from build123d import *

# Parameters (mm, degrees)
SKETCH_1_W          = 60
SKETCH_1_H          = 32
EXTRUDE_1_DEPTH     = 180
SKETCH_2_W          = 56
SKETCH_2_H          = 26
CUT_EXTRUDE_1_DEPTH = 30


with BuildPart() as part:
    # 草图1 → 凸台-拉伸1 (new body)
    with BuildSketch(Plane.XY):
        with Locations((30, 16)):
            Rectangle(SKETCH_1_W, SKETCH_1_H)
    extrude(amount=EXTRUDE_1_DEPTH)

    # 草图2 → 切除-拉伸1 (cut)
    with BuildSketch(Plane(origin=(0, 0, 0), x_dir=(-1, 0, 0), z_dir=(0, -1, 0))):
        with Locations((-30, -165)):
            Rectangle(SKETCH_2_W, SKETCH_2_H)
        with Locations((-30, -135.5)):
            Rectangle(SKETCH_2_W, SKETCH_2_H)
        with Locations((-30, -106)):
            Rectangle(SKETCH_2_W, SKETCH_2_H)
        with Locations((-30, -76.5)):
            Rectangle(SKETCH_2_W, SKETCH_2_H)
        with Locations((-30, -47)):
            Rectangle(SKETCH_2_W, SKETCH_2_H)
        with Locations((-30, -17.5)):
            Rectangle(SKETCH_2_W, SKETCH_2_H)
    extrude(amount=-CUT_EXTRUDE_1_DEPTH, mode=Mode.SUBTRACT)


solid = part.part
Build history of the part. All positions in model axes, mm. A direction names the side the tool comes from. Give positions to 0.01 mm unless a question says otherwise; leave off trailing zeros. Order: outer loops, then holes, each group sorted by start corner. A loop starts at its lowest first (then second) coordinate and runs counter-clockwise, first axis right, second up. Notation, with made-up numbers: M 48.25,46 L 60.25,46 A34 ccw 60.25,84 Z; hole C 1.5,2 d1. An arc over 180 degrees is marked long. Put each result on its own line as item: value.
Item 1: Cut at C-C on x = 13. Write the cut outline in (y, z), then the cut area to 3 significant figures.
Results are:
outline: M 0,0 L 32,0 L 32,180 L 0,180 L 0,178 L 30,178 L 30,152 L 0,152 L 0,148.5 L 30,148.5 L 30,122.5 L 0,122.5 L 0,119 L 30,119 L 30,93 L 0,93 L 0,89.5 L 30,89.5 L 30,63.5 L 0,63.5 L 0,60 L 30,60 L 30,34 L 0,34 L 0,30.5 L 30,30.5 L 30,4.5 L 0,4.5 Z
area: 1,080 mm2
Item 2: Cut at A-A on z = 162. Write the cut outline in (x, y).
Results are:
outline: M 0,0 L 2,0 L 2,30 L 58,30 L 58,0 L 60,0 L 60,32 L 0,32 Z
Item 3: Drop flat-ended pins along their axis: pin 1 Ø6 at (x, y) = (17.5, 7.5) entering from -Z; pin 2 Ø21 at (x, z) = (19.5, 107) entering from -Y. Give the stop position or say it passes through.
Results are:
pin 1: z = 0
pin 2: y = 30
Item 4: Wall check: probe 1 along X at (y, z) = (18, 70); probe 2 along Y at (x, z) = (12.5, 155). Give the ranges that are in metal, low to high.
Results are:
probe 1: 0 to 2, 58 to 60
probe 2: 30 to 32
Item 5: Cut at B-B on y = 5.5. Write the cut outline in (x, z), then the cut area to 3 significant figures.
Results are:
outline: M 0,0 L 60,0 L 60,180 L 0,180 Z; hole M 2,4.5 L 58,4.5 L 58,30.5 L 2,30.5 Z; hole M 2,34 L 58,34 L 58,60 L 2,60 Z; hole M 2,63.5 L 58,63.5 L 58,89.5 L 2,89.5 Z; hole M 2,93 L 58,93 L 58,119 L 2,119 Z; hole M 2,122.5 L 58,122.5 L 58,148.5 L 2,148.5 Z; hole M 2,152 L 58,152 L 58,178 L 2,178 Z
area: 2,060 mm2
Item 6: Which spindle directions (+Z, -Z, +X, -X, +Y, -Y) get a long thin tool onto all of the face, cutting with end or side? Do faces 1 (the face through (58, 15, 77)), 2 (the face through (30, 16, 180)). Say none if no direction does.
Results are:
face 1: -Y
face 2: +Z, +X, -X, +Y, -Y
